from build123d import *

# Parameters (mm, degrees)
BOSS_EXTRUDE1_DEPTH = 60
SKETCH2_W           = 39
SKETCH2_H           = 5.5
BOSS_EXTRUDE2_DEPTH = 8
FILLET2_R           = 2
SKETCH3_W           = 6
SKETCH3_H           = 15
BOSS_EXTRUDE3_DEPTH = 12
SKETCH4_W           = 19
SKETCH4_H           = 15
BOSS_EXTRUDE4_DEPTH = 13
FILLET3_R           = 2
SKETCH5_R           = 2.5
CUT_EXTRUDE1_DEPTH  = 65.439894475


# Some blends are built 0.0001 mm under size
with BuildPart() as part:
    # Sketch1 → Boss-Extrude1 (new body)
    with BuildSketch(Plane.XY):
        Polygon((-26, 0), (26, 0), (26, -5.5), (19.5, -5.5), (19.5, -12.5), (-19.5, -12.5), (-19.5, -5.5), (-26, -5.5), align=None)
    extrude(amount=BOSS_EXTRUDE1_DEPTH)

    # Sketch2 → Boss-Extrude2 (add)
    with BuildSketch(Plane.XY.offset(60)):
        with Locations((0, -2.75)):
            Rectangle(SKETCH2_W, SKETCH2_H)
    extrude(amount=BOSS_EXTRUDE2_DEPTH)

    # Fillet2
    # the kernel refuses this fillet: 2 mm, written as the material it adds along each edge
    with BuildSketch(Plane(origin=(-19.5, 0, 60), x_dir=(-1, 0, 0), z_dir=(0, -1, 0)), Plane(origin=(19.5, -5.5, 60), x_dir=(1, 0, 0), z_dir=(0, 1, 0))) as fillet2_piece_1:
        with BuildLine():
            CenterArc((FILLET2_R, -FILLET2_R), FILLET2_R, 90, 90)
            Line((0, -FILLET2_R), (0, 0))
            Line((0, 0), (FILLET2_R, 0))
        make_face()
    extrude(amount=5.5)
    # the kernel refuses this fillet: 2 mm, written as the material it takes off along each edge
    with BuildSketch(Plane(origin=(26, 5, 60), x_dir=(-1, 0, 0), z_dir=(0, -1, 0)), Plane(origin=(-19.5, 5, 68), x_dir=(0, 0, -1), z_dir=(0, -1, 0)), Plane(origin=(-26, -10.5, 0), x_dir=(0, 0, 1), z_dir=(0, 1, 0)), Plane(origin=(26, 5, 0), x_dir=(0, 0, 1), z_dir=(0, -1, 0))) as fillet2_2_piece_1:
        with BuildLine():
            CenterArc((FILLET2_R, FILLET2_R), FILLET2_R, 180, 90)
            Line((0, FILLET2_R), (0, 0))
            Line((0, 0), (FILLET2_R, 0))
        make_face()
    extrude(amount=15.5, mode=Mode.SUBTRACT)
    with BuildSketch(Plane(origin=(-26, -10.5, 60), x_dir=(0, 0, -1), z_dir=(0, 1, 0)), Plane(origin=(19.5, -10.5, 68), x_dir=(-1, 0, 0), z_dir=(0, 1, 0))) as fillet2_2_piece_2:
        with BuildLine():
            CenterArc((FILLET2_R, -FILLET2_R), FILLET2_R, 90, 90)
            Line((0, -FILLET2_R), (0, 0))
            Line((0, 0), (FILLET2_R, 0))
        make_face()
    extrude(amount=15.5, mode=Mode.SUBTRACT)

    # Sketch3 → Boss-Extrude3 (add)
    with BuildSketch(Plane.XZ.offset(12.5)):
        with Locations((0, 38)):
            Rectangle(SKETCH3_W, SKETCH3_H)
    extrude(amount=BOSS_EXTRUDE3_DEPTH)

    # Sketch4 → Boss-Extrude4 (add)
    with BuildSketch(Plane.XZ.offset(24.5)):
        with Locations((-2.5, 38)):
            Rectangle(SKETCH4_W, SKETCH4_H)
    extrude(amount=BOSS_EXTRUDE4_DEPTH)

    # Fillet3
    fillet3_edges = [part.edges().sort_by_distance(p)[0] for p in [
        (7, -24.5, 38),
        (-12, -24.5, 38),
        (7, -37.5, 38),
        (-12, -37.5, 38),
        (3, -24.5, 38),
        (-3, -24.5, 38),
    ]]
    fillet(fillet3_edges, radius=FILLET3_R - 0.0001)  # a hair under: the kernel refuses the full size

    # Sketch5 → Cut-Extrude1 (cut, through all)
    with BuildSketch(Plane.XY.offset(45.5)):
        with Locations((0, -31)):
            Circle(SKETCH5_R)
    extrude(amount=-CUT_EXTRUDE1_DEPTH, mode=Mode.SUBTRACT)


solid = part.part
Verification items for the finished model (mm, model axes). A direction names the side the tool comes from. Coordinates: 2 decimals unless noted, no trailing zeros. Order: outer loops, then holes, each group sorted by start corner. A loop starts at its lowest first (then second) coordinate and runs counter-clockwise, first axis right, second up.
Item 1: Section check D-D, the plane x = 16. Enter the section's corners in (y, z).
Filled in:
outline: (-12.5, 0) - (0, 0) - (0, 68) - (-5.5, 68) - (-5.5, 60) - (-12.5, 60) - close
Item 2: Access from +Z, -Z, +X, -X, +Y, -Y to the whole of each face (thin tool, end or side, straight path). Record for faces 1 (the face through (19.5, -3, 64)), 2 (the face through (3.6, -23.93, 38.11)), 3 (the face through (-3, -28, 30.5)), 4 (the face through (19.5, -9, 30)), 5 (the face through (-19.5, -3, 64)).
Filled in:
face 1: +Z, +X, +Y, -Y
face 2: +Z, -Z, +X
face 3: -Z, +X, -X, -Y
face 4: +Z, -Z, +X, -Y
face 5: +Z, -X, +Y, -Y
Item 3: Material ranges on L1, parallel to Y at x = 0, z = 34.75; L2, parallel to Y at x = 0, z = 23.5; L3, parallel to Z at x = 24, y = -3, recorded low to high.
Filled in:
L1: y = -37.5 to -33.5, -28.5 to 0
L2: y = -12.5 to 0
L3: z = 0 to 60
Item 4: Section check B-B, the plane y = -31. Enter the section's corners in (x, z), then the cut area to 3 significant figures.
Filled in:
outline: (-12, 30.5) - (-2.5, 30.5) - (-2.5, 45.5) - (-12, 45.5) - close; (2.5, 30.5) - (7, 30.5) - (7, 45.5) - (2.5, 45.5) - close
area: 210 mm2
Item 5: Depth check by flat-ended pin: pin 1 (8 mm diameter, centred on y = -19.5, z = 35.5, fed in from -X); pin 2 (3 mm diameter, centred on y = -19.5, z = 35.5, fed in from +X); pin 3 (4.5 mm diameter, centred on y = -30, z = 40, fed in from -X); pin 4 (5.5 mm diameter, centred on x = -7, y = -20.5, fed in from -Z). Enter the tip coordinate at first touch or a pass-through.
Filled in:
pin 1: stops at x = -3.27
pin 2: stops at x = 3
pin 3: stops at x = -12
pin 4: passes through
Item 6: Release check for a two-part mould opening along X. For faces 6 (the face through (-8, -24.5, 38)), 7 (the face through (-0.33, -28.52, 38.11)), 8 (the face through (-11.43, -36.9, 38.11)) record: +X half, -X half, draft (parallel to the pull), parting line (faces both ways), or undercut.
Filled in:
face 6: draft
face 7: undercut
face 8: -X half
Item 7: Section check A-A, the plane x = 0. Enter the section's corners in (y, z).
Filled in:
outline: (-37.5, 30.5) - (-33.5, 30.5) - (-33.5, 45.5) - (-37.5, 45.5) - close; (-28.5, 30.5) - (-12.5, 30.5) - (-12.5, 0) - (0, 0) - (0, 68) - (-5.5, 68) - (-5.5, 60) - (-12.5, 60) - (-12.5, 45.5) - (-28.5, 45.5) - close
Item 8: Section check C-C, the plane z = 51. Enter the section's corners in (x, y), then the cut area to 3 significant figures.
Filled in:
outline: (-26, -5.5) - (-19.5, -5.5) - (-19.5, -12.5) - (19.5, -12.5) - (19.5, -5.5) - (26, -5.5) - (26, 0) - (-26, 0) - close
area: 559 mm2
